CAD build for the part. Positions are in the model's coordinates, mm. A direction names the side the tool comes from. Coordinates: 2 decimals unless noted, no trailing zeros. Loops run counter-clockwise (first coordinate to the right, second up) from the corner with the lowest first, then second, coordinate; pieces in that order, holes last. Notation, with made-up numbers: M 78,13 L 132,13 A18 cw 132,47 Z; hole C 89.5,-5.75 d8. An arc over 180 degrees is marked long. Answer as a JSON object with one key per item and string values. Group by question number.
```python
from build123d import *

# Parameters (mm, degrees)
BOSS_EXTRUDE1_DEPTH      = 3.81
LPATTERN1_COUNT          = 2
LPATTERN1_PITCH          = 61
BODY_MOVE_COPY1_ANGLE    = 180
LPATTERN2_COUNT          = 3
LPATTERN2_PITCH          = 146.05
BODY_MOVE_COPY2_ANGLE    = 120
BODY_MOVE_COPY3_ANGLE    = 120
BOSS_EXTRUDE2_START      = 59.53
SKETCH2_R                = 9.5
BOSS_EXTRUDE2_DEPTH      = 1
BOSS_EXTRUDE2_DEPTH_BACK = 466.09


with BuildPart() as part:
    # Sketch1 → Boss-Extrude1 (new body, symmetric)
    with BuildSketch(Plane(origin=(0, 0, 0), x_dir=(1, 0, 0), z_dir=(0, 1, 0))):
        with BuildLine():
            Line((-5.499261314, 15.875), (-10.998522628, 6.35))
            ThreePointArc((-10.998522628, 6.35), (0, -12.7), (10.998522628, 6.35))
            Line((10.998522628, 6.35), (5.499261314, 15.875))
            ThreePointArc((5.499261314, 15.875), (0, 19.05), (-5.499261314, 15.875))
        make_face()
    extrude(amount=BOSS_EXTRUDE1_DEPTH, both=True)


with BuildPart() as lpattern1_1:
    # LPattern1: pattern copy
    add(part.part.moved(Location(Vector(0, -1, 0) * (1 * LPATTERN1_PITCH))))


with BuildPart() as lpattern1_1_1:
    # Body-Move_Copy1: moved
    add(lpattern1_1.part.rotate(Axis((0, 0, 0), (0, 1, 0)), BODY_MOVE_COPY1_ANGLE))


with BuildPart() as lpattern2_1:
    # LPattern2: pattern copy
    add(part.part.moved(Location(Vector(0, -1, 0) * (1 * LPATTERN2_PITCH))))


with BuildPart() as lpattern2_2:
    # LPattern2: pattern copy
    add(part.part.moved(Location(Vector(0, -1, 0) * (2 * LPATTERN2_PITCH))))


with BuildPart() as lpattern2_3:
    # LPattern2: pattern copy
    add(lpattern1_1_1.part.moved(Location(Vector(0, -1, 0) * (1 * LPATTERN2_PITCH))))


with BuildPart() as lpattern2_4:
    # LPattern2: pattern copy
    add(lpattern1_1_1.part.moved(Location(Vector(0, -1, 0) * (2 * LPATTERN2_PITCH))))


with BuildPart() as lpattern2_1_1:
    # Body-Move_Copy2: moved
    add(lpattern2_1.part.rotate(Axis((0, 0, 0), (0, -1, 0)), BODY_MOVE_COPY2_ANGLE))


with BuildPart() as lpattern2_3_1:
    # Body-Move_Copy2: moved
    add(lpattern2_3.part.rotate(Axis((0, 0, 0), (0, -1, 0)), BODY_MOVE_COPY2_ANGLE))


with BuildPart() as lpattern2_2_1:
    # Body-Move_Copy3: moved
    add(lpattern2_2.part.rotate(Axis((0, 0, 0), (0, 1, 0)), BODY_MOVE_COPY3_ANGLE))


with BuildPart() as lpattern2_4_1:
    # Body-Move_Copy3: moved
    add(lpattern2_4.part.rotate(Axis((0, 0, 0), (0, 1, 0)), BODY_MOVE_COPY3_ANGLE))


with BuildPart() as part_1:
    add(part.part)

    add(lpattern1_1_1.part)  # Boss-Extrude2 merges LPattern1_1

    add(lpattern2_1_1.part)  # Boss-Extrude2 merges LPattern2_1

    add(lpattern2_2_1.part)  # Boss-Extrude2 merges LPattern2_2

    add(lpattern2_3_1.part)  # Boss-Extrude2 merges LPattern2_3

    add(lpattern2_4_1.part)  # Boss-Extrude2 merges LPattern2_4
    # Sketch2 → Boss-Extrude2 (add, two sides)
    with BuildSketch(Plane(origin=(0, 0, 0), x_dir=(1, 0, 0), z_dir=(0, 1, 0)).offset(BOSS_EXTRUDE2_START)) as boss_extrude2_sk:
        Circle(SKETCH2_R)
    extrude(amount=BOSS_EXTRUDE2_DEPTH)
    extrude(boss_extrude2_sk.sketch, amount=-BOSS_EXTRUDE2_DEPTH_BACK)


solid = part_1.part
```
Item 1: Pull direction Y, two halves, no side cores. Call faces 1 (the cylindrical face through (4.38, -30.13, 8.43)), 2 (the flat face through (-13.8, -207, 1.5)): released by +Y, released by -Y, zero draft, split by the parting line, or undercut.
Item 2: Drill centre lines: L1, parallel to Y at x = 11.5, z = -5; L2, parallel to Z at x = 0.5, y = -14; L3, parallel to X at y = -129, z = -1. Where is each one in solid material? Low to high. Write a range as from..to.
Item 3: Slice it at A-A, the plane y = -244. Write the cut outline in (x, z).
Item 4: Pin check, flat tips, straight feed: pin 1 (1.5 mm diameter, centred on y = -170, z = 4.5, fed in from +X); pin 2 (1 mm diameter, centred on x = -8.5, y = 3.5, fed in from +Z); pin 3 (1.5 mm diameter, centred on x = 7.5, y = -239, fed in from -Z); pin 4 (3 mm diameter, centred on x = 6, z = 7.5, fed in from -Y). Stop position of each tip, or through.
Item 5: Tool access for faces 3 (the flat face through (-9, -288.29, 4)), 4 (the flat face through (13.71, -353.05, 1.65)), 5 (the flat face through (-5, -207, -12.7)), 6 (the flat face through (8.287, 0.053, -11.046)), 7 (the flat face through (-8.287, -60.947, 11.046)): list every direction of +Z, -Z, +X, -X, +Y, -Y with a clear straight run to the whole face (end or side of a thin tool).
Computed:
{
 "1": {"face 1": "undercut", "face 2": "zero draft"},
 "2": {"L1": "-356.91..-349.29, -295.91..-288.29, -210.86..-203.24, -149.86..-142.24, -64.81..-57.19, -3.81..3.81", "L2": "-9.49..9.49", "L3": "-9.45..9.45"},
 "3": {"outline": "C 0,0 d19"},
 "4": {"pin 1": "x = 8.73", "pin 2": "z = 9.86", "pin 3": "z = -6.68", "pin 4": "y = -406.56"},
 "5": {"face 3": "none", "face 4": "+Z, +X, -Y", "face 5": "-Z, +X, -X, -Y", "face 6": "-Z, +X, +Y", "face 7": "+Z, -X, +Y"}
}
